Design review of the part built by this model. Coordinates are the model's own, in mm. Face numbers are marked on the shaded views. A direction names the side the tool comes from. Round coordinates to 2 decimals unless told otherwise and drop trailing zeros. Loops run counter-clockwise (first coordinate to the right, second up) from the corner with the lowest first, then second, coordinate; pieces in that order, holes last. Notation, with made-up numbers: M 6.25,73.25 L 62.25,73.25 A16 ccw 62.25,89.25 Z; hole C 26.25,-29 d4. An arc over 180 degrees is marked long. One line per item, written item: value. Start each with the question number.
Item 1: We need section A-A (x = 64.5). Write out the cut boundary in (y, z), then the cut area to 3 significant figures.
Item 2: Mouldability with a two-part tool opening along X and no side actions: class the marked faces 1, 2 and 3 as released by +X, released by -X, zero draft, split by the parting line, or undercut.
Item 3: Clearance check with flat-ended pins moving along their axes: pin 1 (8.5 mm diameter, centred on x = 2.5, z = 17.5, fed in from +Y); pin 2 (1.5 mm diameter, centred on y = 3, z = 31, fed in from -X); pin 3 (3 mm diameter, centred on x = 9.5, z = 10, fed in from +Y); pin 4 (4 mm diameter, centred on x = 11, y = 0, fed in from -Z). State where each tip first meets the part, or that it passes through.
Item 4: We need section B-B (y = -1.25). Write out the cut boundary in (x, z), then the cut area to 3 significant figures.
Item 5: We need section C-C (x = 17.5). Write out the cut boundary in (y, z), then the cut area to 3 significant figures.
Item 6: For the marked faces 4, 5 and 6, list the 3-axis set-ups (+Z, -Z, +X, -X, +Y, -Y) from which the entire face can be reached by the end or side of a thin tool; tool diameter is ignored.
Item 7: For line 1 along Y through (x, z) = (20, 45); line 2 along X through (y, z) = (3, 9); line 3 along Z through (x, y) = (46.5, 1.5), list the stretches that pass through material, from the lowest coordinate up.
from build123d import *

# Parameters (mm, degrees)
F1_DEPTH    = 50
F2_SIZE2    = 2.99999
F2_SIZE     = 49.99999
F3_T1_DEPTH = 57.5899085645
F4_R        = 2
F5_R        = 3
F6_W        = 9
F6_H        = 5
F7_DEPTH    = 75
F8_R        = 2


# Not quite as in the source:
# - a fillet or chamfer that OpenCascade refuses, or shapes differently, is made with other operations: its cross-section is extruded or revolved along the edge and cut away or added
# - a fillet or chamfer is up to 0.001 mm smaller than in the source, because OpenCascade refuses the exact size


with BuildPart() as f1:
    # F0 (on Top) → F1 (new body)
    with BuildSketch(Plane.XY):
        Polygon((-4.3715766435, 7.6504380477), (-7.7186432894, 6.6271370812), (-4.4696014276, -4), (20.5303985724, -4), (20.5303985724, 5), (8.0088521886, 5), (6.9673969943, 0), (-2.0326030057, 0), align=None)
    extrude(amount=F1_DEPTH)

    # F2 (size 50 and 3 in the source; OpenCascade refuses exactly that, so slightly less here)
    f2_edges = [f1.edges().sort_by_distance(p)[0] for p in [
        (-6.04511, 7.138788, 0),
    ]]
    f2_side = f1.faces().sort_by_distance((-6.04511, 7.138788, 25))[0]
    chamfer(f2_edges, length=F2_SIZE, length2=F2_SIZE2, reference=f2_side)

    # F3: fillet of radius 1.5 on 2 edges, made by hand

    # F3_s2 → F3_t1 (cut)
    with BuildSketch(Plane(origin=(-0.948644568, 3.1028765694, 54.0777102773), x_dir=(0.956304756, 0.2923717047, 0), z_dir=(0.0175107565, -0.0572751036, -0.9982048567))):
        with BuildLine():
            ThreePointArc((-1.9437879213, -4.0842430614), (-2.3831277496, -5.1449032332), (-3.4437879213, -5.5842430614))
            Line((-3.4437879213, -5.5842430614), (-1.9437879213, -5.5842430614))
            Line((-1.9437879213, -5.5842430614), (-1.9437879213, -4.0842430614))
        make_face()
        with BuildLine():
            ThreePointArc((-3.9437879213, -5.5842430614), (-5.0044480931, -5.1449032332), (-5.4437879213, -4.0842430614))
            Line((-5.4437879213, -4.0842430614), (-5.4437879213, -5.5842430614))
            Line((-5.4437879213, -5.5842430614), (-3.9437879213, -5.5842430614))
        make_face()
    extrude(amount=F3_T1_DEPTH, mode=Mode.SUBTRACT)

    # F4
    f4_edges = [f1.edges().sort_by_distance(p)[0] for p in [
        (-2.032603, 0, 25),
    ]]
    fillet(f4_edges, radius=F4_R)

    # F5
    f5_edges = [f1.edges().sort_by_distance(p)[0] for p in [
        (8.008852, 5, 25),
    ]]
    fillet(f5_edges, radius=F5_R)

    # F6 (on face) → F7 (join)
    with BuildSketch(Plane.YZ.offset(20.5303985724)):
        with Locations((0.5, 47.5)):
            Rectangle(F6_W, F6_H)
    extrude(amount=F7_DEPTH)

    # F8
    f8_edges = [f1.edges().sort_by_distance(p)[0] for p in [
        (-4.469601, -4, 25),
    ]]
    fillet(f8_edges, radius=F8_R)


solid = f1.part
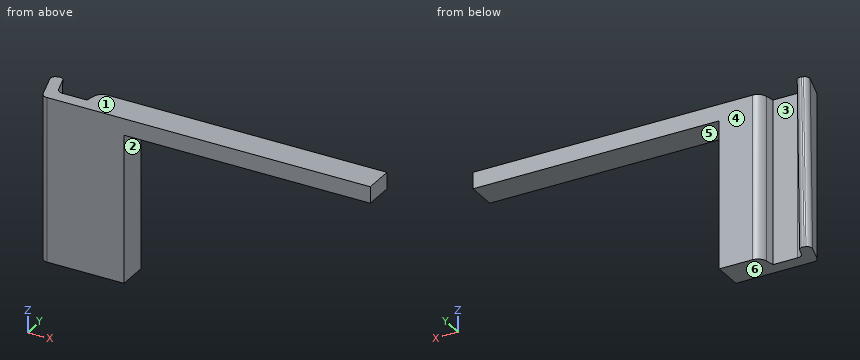
A:
1. outline: M -4,45 L 5,45 L 5,50 L -4,50 Z
1. area: 45.0 mm2
2. face 1: zero draft
2. face 2: released by +X
2. face 3: undercut
3. pin 1: y = 0.4
3. pin 2: x = -6.84
3. pin 3: y = 5
3. pin 4: z = 0
4. outline: M -5.31,0 L 20.53,0 L 20.53,45 L 95.53,45 L 95.53,50 L -5.31,50 Z
4. area: 1,670 mm2
5. outline: M -4,0 L 5,0 L 5,50 L -4,50 Z
5. area: 450 mm2
6. face 4: +Z, -Z, +X, +Y
6. face 5: -Z, +X, +Y, -Y
6. face 6: -Z, +X, -X, +Y, -Y
7. line 1: -4 to 5
7. line 2: -6.6 to -2.95, 7.62 to 20.53
7. line 3: 45 to 50
